Source: three-view drawing plus pictorial views. Frame: mm from the lowest corner of the part. Give positions to 0.01 mm unless a question says otherwise; leave off trailing zeros. Loops run counter-clockwise (first coordinate to the right, second up) from the corner with the lowest first, then second, coordinate; pieces in that order, holes last. Notation, with made-up numbers: (48, 86) - (55, 86) arc R16 cw to (55, 115) - close; hole circle Ø7 at (48.25, -6). An arc over 180 degrees is marked (long way). One line per item, written item: value.
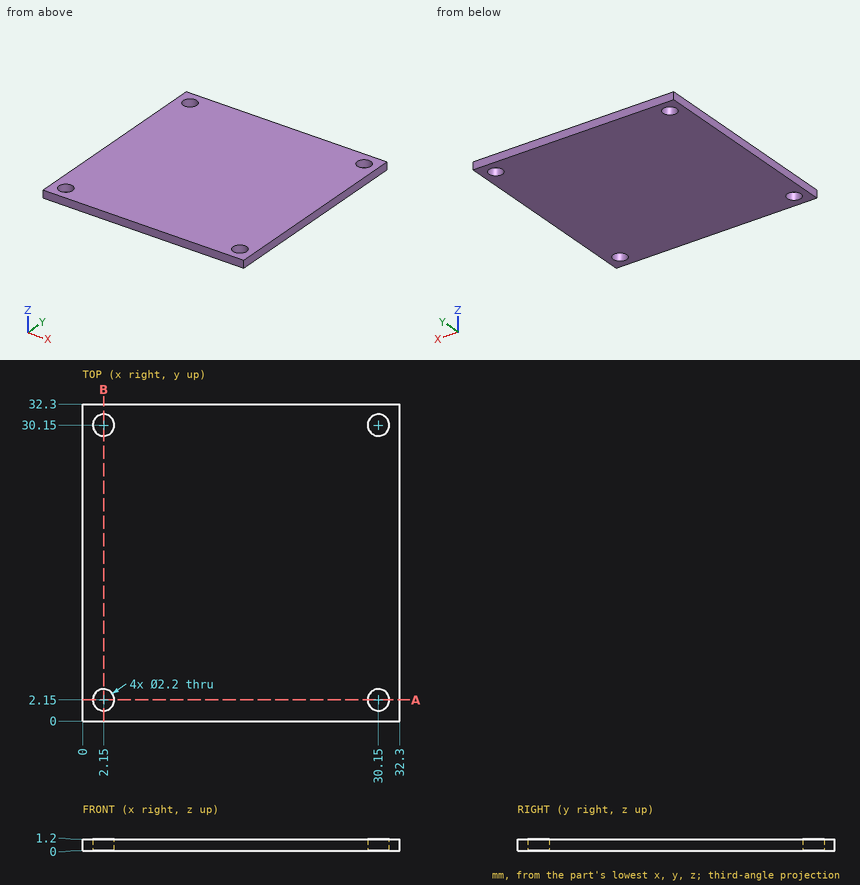
Item 1: Material intervals for L1, parallel to Y at x = 2.15, z = 0.9; L2, parallel to X at y = 3, z = 0.75, sorted ascending.
Verdict:
L1: y = 0 to 1.05, 3.25 to 29.05, 31.25 to 32.3
L2: x = 0 to 1.45, 2.85 to 29.45, 30.85 to 32.3
Item 2: Section A-A, the plane y = 2.15. Output: boundary loops of the cut face in (x, z), and give its area (3 significant figures).
Verdict:
outline: (0, 0) - (1.05, 0) - (1.05, 1.2) - (0, 1.2) - close; (3.25, 0) - (29.05, 0) - (29.05, 1.2) - (3.25, 1.2) - close; (31.25, 0) - (32.3, 0) - (32.3, 1.2) - (31.25, 1.2) - close
area: 33.5 mm^2
